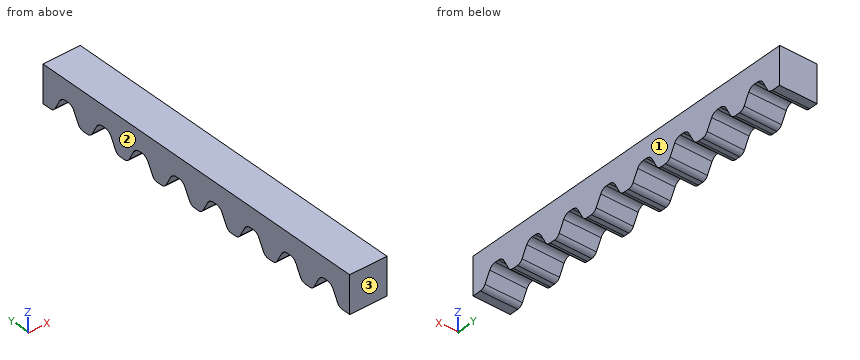
from build123d import *

# Parameters (mm, degrees)
RACK_DEPTH = 30


with BuildPart() as part:
    # Sketch1 → RACK (new body)
    with BuildSketch(Plane(origin=(0, 0, 0), x_dir=(0, 0, -1), z_dir=(1, 0, 0))):
        with BuildLine():
            Line((0, 0), (0, -290))
            Line((0, -290), (30, -290))
            Line((30, -290), (30, -282.993707205))
            ThreePointArc((30, -282.993707205), (29.289844712, -280.4251994), (27.361107063, -278.586307355))
            Line((27.361107063, -278.586307355), (19.166671525, -274.196431174))
            ThreePointArc((19.166671525, -274.196431174), (16.852186345, -271.98976072), (16, -268.907551354))
            Line((16, -268.907551354), (16, -266.092448646))
            ThreePointArc((16, -266.092448646), (16.852186345, -263.01023928), (19.166671525, -260.803568826))
            Line((19.166671525, -260.803568826), (27.361107063, -256.413692645))
            ThreePointArc((27.361107063, -256.413692645), (29.289844712, -254.5748006), (30, -252.006292795))
            Line((30, -252.006292795), (30, -247.993707205))
            ThreePointArc((30, -247.993707205), (29.289844712, -245.4251994), (27.361107063, -243.586307355))
            Line((27.361107063, -243.586307355), (19.166671525, -239.196431174))
            ThreePointArc((19.166671525, -239.196431174), (16.852186345, -236.98976072), (16, -233.907551354))
            Line((16, -233.907551354), (16, -231.092448646))
            ThreePointArc((16, -231.092448646), (16.852186345, -228.01023928), (19.166671525, -225.803568826))
            Line((19.166671525, -225.803568826), (27.361107063, -221.413692645))
            ThreePointArc((27.361107063, -221.413692645), (29.289844712, -219.5748006), (30, -217.006292795))
            Line((30, -217.006292795), (30, -212.993707205))
            ThreePointArc((30, -212.993707205), (29.289844712, -210.4251994), (27.361107063, -208.586307355))
            Line((27.361107063, -208.586307355), (19.166671525, -204.196431174))
            ThreePointArc((19.166671525, -204.196431174), (16.852186345, -201.98976072), (16, -198.907551354))
            Line((16, -198.907551354), (16, -196.092448646))
            ThreePointArc((16, -196.092448646), (16.852186345, -193.01023928), (19.166671525, -190.803568826))
            Line((19.166671525, -190.803568826), (27.361107063, -186.413692645))
            ThreePointArc((27.361107063, -186.413692645), (29.289844712, -184.5748006), (30, -182.006292795))
            Line((30, -182.006292795), (30, -177.993707205))
            ThreePointArc((30, -177.993707205), (29.289844712, -175.4251994), (27.361107063, -173.586307355))
            Line((27.361107063, -173.586307355), (19.166671525, -169.196431174))
            ThreePointArc((19.166671525, -169.196431174), (16.852186345, -166.98976072), (16, -163.907551354))
            Line((16, -163.907551354), (16, -161.092448646))
            ThreePointArc((16, -161.092448646), (16.852186345, -158.01023928), (19.166671525, -155.803568826))
            Line((19.166671525, -155.803568826), (27.361107063, -151.413692645))
            ThreePointArc((27.361107063, -151.413692645), (29.289844712, -149.5748006), (30, -147.006292795))
            Line((30, -147.006292795), (30, -142.993707205))
            ThreePointArc((30, -142.993707205), (29.289844712, -140.4251994), (27.361107063, -138.586307355))
            Line((27.361107063, -138.586307355), (19.166671525, -134.196431174))
            ThreePointArc((19.166671525, -134.196431174), (16.852186345, -131.98976072), (16, -128.907551354))
            Line((16, -128.907551354), (16, -126.092448646))
            ThreePointArc((16, -126.092448646), (16.852186345, -123.01023928), (19.166671525, -120.803568826))
            Line((19.166671525, -120.803568826), (27.361107063, -116.413692645))
            ThreePointArc((27.361107063, -116.413692645), (29.289844712, -114.5748006), (30, -112.006292795))
            Line((30, -112.006292795), (30, -107.993707205))
            ThreePointArc((30, -107.993707205), (29.289844712, -105.4251994), (27.361107063, -103.586307355))
            Line((27.361107063, -103.586307355), (19.166671525, -99.196431174))
            ThreePointArc((19.166671525, -99.196431174), (16.852186345, -96.98976072), (16, -93.907551354))
            Line((16, -93.907551354), (16, -91.092448646))
            ThreePointArc((16, -91.092448646), (16.852186345, -88.01023928), (19.166671525, -85.803568826))
            Line((19.166671525, -85.803568826), (27.361107063, -81.413692645))
            ThreePointArc((27.361107063, -81.413692645), (29.289844712, -79.5748006), (30, -77.006292795))
            Line((30, -77.006292795), (30, -72.993707205))
            ThreePointArc((30, -72.993707205), (29.289844712, -70.4251994), (27.361107063, -68.586307355))
            Line((27.361107063, -68.586307355), (19.166671525, -64.196431174))
            ThreePointArc((19.166671525, -64.196431174), (16.852186345, -61.98976072), (16, -58.907551354))
            Line((16, -58.907551354), (16, -56.092448646))
            ThreePointArc((16, -56.092448646), (16.852186345, -53.01023928), (19.166671525, -50.803568826))
            Line((19.166671525, -50.803568826), (27.361107063, -46.413692645))
            ThreePointArc((27.361107063, -46.413692645), (29.289844712, -44.5748006), (30, -42.006292795))
            Line((30, -42.006292795), (30, -37.993707205))
            ThreePointArc((30, -37.993707205), (29.289844712, -35.4251994), (27.361107063, -33.586307355))
            Line((27.361107063, -33.586307355), (19.166671525, -29.196431174))
            ThreePointArc((19.166671525, -29.196431174), (16.852186345, -26.98976072), (16, -23.907551354))
            Line((16, -23.907551354), (16, -21.092448646))
            ThreePointArc((16, -21.092448646), (16.852186345, -18.01023928), (19.166671525, -15.803568826))
            Line((19.166671525, -15.803568826), (27.361107063, -11.413692645))
            ThreePointArc((27.361107063, -11.413692645), (29.289844712, -9.5748006), (30, -7.006292795))
            Line((30, -7.006292795), (30, 0))
            Line((30, 0), (0, 0))
        make_face()
    extrude(amount=RACK_DEPTH)


solid = part.part
Verification items for the finished model (mm, model axes). Face numbers are marked on the shaded views. Coordinates: 2 decimals unless noted, no trailing zeros. Put each result on its own line as item: value. Start each with the question number.
1. Cross-section at A-A, the plane z = -23. Count the separate pieces of the cut face and the enclosed holes in it, then the cut area to 3 significant figures.
2. Material ranges on L1, parallel to Z at x = 6.5, y = -160.5; L2, parallel to Z at x = 9.25, y = -50, recorded low to high. Write a range as [from, to].
3. Go/stop test with flat-tipped pins: pin 1 Ø2.5 at (x, y) = (11, -233) entering from -Z; pin 2 Ø1.5 at (x, y) = (4.5, -94) entering from -Z. Record where each tip stops, or that it passes through.
4. Mould release check, pull along X, two halves, no side actions. Record for the marked faces 1, 2 and 3: released by +X, released by -X, zero draft, split by the parting line, or undercut.
Computed:
1. separate pieces: 9
1. enclosed holes: 0
1. area: 4,500 mm2
2. L1: [-16.03, 0]
2. L2: [-20.67, 0]
3. pin 1: z = -16.01
3. pin 2: z = -16.06
4. face 1: released by +X
4. face 2: released by -X
4. face 3: zero draft
